Source: CAD feature listing. Evaluate the final solid. Frame: model axes, mm. Face numbers are marked on the shaded views. A direction names the side the tool comes from. Round coordinates to 2 decimals unless told otherwise and drop trailing zeros. Loops run counter-clockwise (first coordinate to the right, second up) from the corner with the lowest first, then second, coordinate; pieces in that order, holes last.
(1) Section B-B, the plane x = -49. Return the cut outline in (y, z).
(2) Section A-A, the plane z = 0. Return the cut outline in (x, y) (3 decimals), plus the area to 3 significant figures.
(3) Set-up query: the marked faces 4 and 5. Return all of +Z, -Z, +X, -X, +Y, -Y with unobstructed straight access to the full face (end or side cutting, diameter ignored); none if empty.
(4) Section D-D, the plane y = 7. Return the cut outline in (x, z).
(5) Mould query, pull axis Z, two halves, no side actions, for the marked faces 1, 2 and 3. Classes: pulls with the +Z half, pulls with the -Z half, needs draft (parallel to the pull), parting line crosses it, or undercut.
(6) Material intervals for probe 1 along X at (y, z) = (1, -1); probe 2 along X at (y, z) = (7.3, 0); probe 3 along Z at (x, y) = (-12, 0.7), sorted ascending.
(7) First-contact query: pin 1 Ø2 at (y, z) = (3.5, 0) entering from +X; pin 2 Ø3.5 at (x, z) = (-40, 0) entering from -Y. Flat tips, straight axial feed; report the tip coordinate or a pass-through.
(8) Section C-C, the plane z = 3.75. Return the cut outline in (x, y) (3 decimals), plus the area to 3 significant figures.
Autodesk Inventor part; units mm, degrees
ref_plane "Work Plane1" through (-52, 11, 4.5) normal (0, 1, 0) x (1, 0, 0)
ref_plane "YZ Plane" through (0, 0, 0) normal (1, 0, 0) x (0, 1, 0)
ref_plane "XZ Plane" through (0, 0, 0) normal (0, 1, 0) x (-1, 0, 0)
sketch "Sketch1" plane through (0, 0, 0) normal (0, 0, 1) x (1, 0, 0)
  line L0 (0, 0) -> (0, 3)
  line L1 (0, 0) -> (0, 40.1132) construction
  arc A0 (-23.165, 3.7081) -> (-20.6, 3) centre (-20.6, 8) ccw
  line L2 (0, 3) -> (-20.6, 3)
  line L3 (0, 0) -> (-20.6, 0)
  arc A1 (-24.704, 1.1329) -> (-20.6, 0) centre (-20.6, 8) ccw
  line L4 (-52, 6) -> (-33.4, 6)
  line L5 (-52, 6) -> (-52, 9)
  line L6 (-52, 9) -> (-33.4, 9)
  circle A2 centre (-33.4, 4) radius 2
  arc A3 (-30.835, 8.2919) -> (-37.9826, 6) centre (-33.4, 4) ccw
  line L7 (-32.374, 5.7168) -> (-24.704, 1.1329)
  line L8 (-30.835, 8.2919) -> (-23.165, 3.7081)
  dimension "d9" = 4
  dimension "d0" = 20.6
  dimension "d2" = 10
  dimension "d3" = 3
  dimension "d4" = 6
  dimension "d5" = 12.8
  dimension "d6" = 3
  dimension "d7" = 18.6
  dimension "d8" = 18.6
  dimension "d10" = 10
  dimension "d11" = 12.8
extrude "Extrusion1" add sketch "Sketch1" along normal mid plane 9 contours L3 A1 L7 A2 L4 A3 L8 A0 L2 L0 | A3 L4 L5 L6
ref_plane "Work Plane1" through (-52, 11, 4.5) normal (0, 1, 0) x (1, 0, 0)
sketch "Sketch2" plane through (-52, 11, 4.5) normal (0, 1, 0) x (1, 0, 0)
  line L0 (0, 9) -> (0, 0)
  line L1 (31.4, 9) -> (52, 9)
  line L2 (18.6, 9) -> (0, 9)
  line L3 (3, 9) -> (3, 0) construction
  line L4 (18.6, 0) -> (0, 0)
  line L5 (12, 9) -> (12, 0) construction
  line L6 (49, 9) -> (49, 0) construction
  line L7 (31.4, 0) -> (52, 0)
  line L8 (0, 4.5) -> (52, 4.5) construction
  line L9 (52, 9) -> (52, 0)
  line L10 (40, 9) -> (40, 0) construction
  circle A0 centre (3, 4.5) radius 1.5
  circle A1 centre (12, 4.5) radius 1.5
  circle A2 centre (40, 4.5) radius 1.5
  circle A3 centre (49, 4.5) radius 1.5
  dimension "d15" = 3
  dimension "d16" = 9
  dimension "d17" = 3
  dimension "d18" = 9
  dimension "d19" = 3
  dimension "d20" = 3
  dimension "d21" = 3
  dimension "d22" = 3
hole "Hole1" at (-12, 11, 0) at (-3, 11, 0) at (-40, 11, 0) at (-49, 11, 0) direction (0, -1, 0) diameter 3 end through all
equation "\"d8\" = d7"
properties part number "Hudson 1-68"
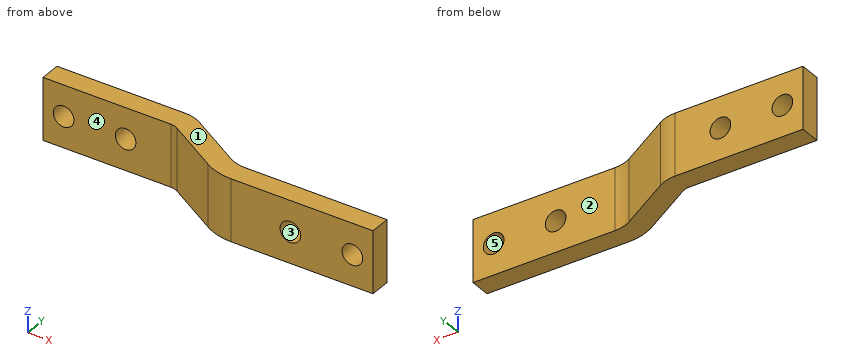
Output values:
1. outline: (6, -4.5) - (9, -4.5) - (9, -1.5) - (6, -1.5) - close; (6, 1.5) - (9, 1.5) - (9, 4.5) - (6, 4.5) - close
2. outline: (-52, 6) - (-50.5, 6) - (-50.5, 9) - (-52, 9) - close; (-47.5, 6) - (-41.5, 6) - (-41.5, 9) - (-47.5, 9) - close; (-38.5, 6) - (-33.4, 6) arc R2 cw to (-32.374, 5.717) - (-24.704, 1.133) arc R8 ccw to (-20.6, 0) - (-13.5, 0) - (-13.5, 3) - (-20.6, 3) arc R5 cw to (-23.165, 3.708) - (-30.835, 8.292) arc R5 ccw to (-33.4, 9) - (-38.5, 9) - close; (-10.5, 0) - (-4.5, 0) - (-4.5, 3) - (-10.5, 3) - close; (-1.5, 0) - (0, 0) - (0, 3) - (-1.5, 3) - close
2. area: 125 mm2
3. face 4: +Z, -Z, -X, -Y
3. face 5: +Y, -Y
4. outline: (-52, -4.5) - (-28.67, -4.5) - (-28.67, 4.5) - (-52, 4.5) - close; hole circle Ø3 at (-49, 0); hole circle Ø3 at (-40, 0)
5. face 1: pulls with the +Z half
5. face 2: needs draft
5. face 3: undercut
6. probe 1: x = -24.47 to -13.12, -10.88 to -4.12, -1.88 to 0
6. probe 2: x = -52 to -50.5, -47.5 to -41.5, -38.5 to -29.18
6. probe 3: z = -4.5 to -1.5, 1.5 to 4.5
7. pin 1: stops at x = 0
7. pin 2: stops at y = 6
8. outline: (-52, 6) - (-33.4, 6) arc R2 cw to (-32.374, 5.717) - (-24.704, 1.133) arc R8 ccw to (-20.6, 0) - (0, 0) - (0, 3) - (-20.6, 3) arc R5 cw to (-23.165, 3.708) - (-30.835, 8.292) arc R5 ccw to (-33.4, 9) - (-52, 9) - close
8. area: 161 mm2
